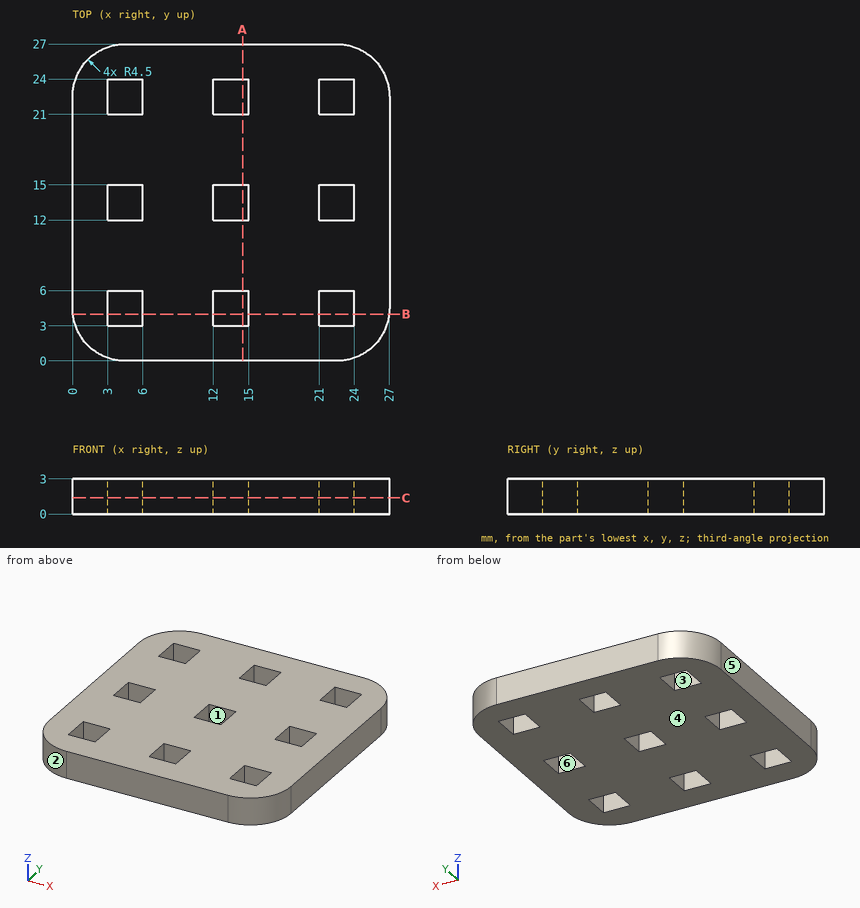
Input: dimensioned drawing with shaded views. Units: mm. Origin: part minimum x, y, z. A direction names the side the tool comes from. Coordinates: 2 decimals unless noted, no trailing zeros. Order: outer loops, then holes, each group sorted by start corner. A loop starts at its lowest first (then second) coordinate and runs counter-clockwise, first axis right, second up. Notation, with made-up numbers: M -37.75,2 L -10.75,2 A21 ccw -10.75,23 Z; hole C -27,-17 d4. An arc over 180 degrees is marked long. Write each question's results on one line, items separated by ' | '. Start each with the question number.
Item 1: First-contact query: pin 1 Ø0.9 at (x, z) = (22, 2) entering from -Y. Flat tip, straight axial feed; report the tip coordinate or a pass-through.
Item 2: Line query: probe 1 along X at (y, z) = (4.5, 1.1); probe 2 along Y at (x, z) = (3.75, 0.2). Output: solid intervals per line, ascending.
Item 3: Cut plane B-B (y = 4). Return loops of the section in (x, z).
Item 4: Cut plane C-C (z = 1.4). Count the separate pieces of the cut face and the enclosed holes in it, and give its area (3 significant figures).
Item 5: Draft query along X for the marked faces 1, 2, 3 and 4. Return one class per face: pulls with the +X half, pulls with the -X half, needs draft (parallel to the pull), parting line crosses it, or undercut.
Item 6: Set-up query: the marked faces 5 and 6. Return all of +Z, -Z, +X, -X, +Y, -Y with unobstructed straight access to the full face (end or side cutting, diameter ignored); none if empty.
Item 7: Cut plane A-A (x = 14.5). Return loops of the section in (y, z), and give its area (3 significant figures).
Checked values:
1) pin 1: stops at y = 0
2) probe 1: x = 0 to 3, 6 to 12, 15 to 21, 24 to 27 | probe 2: y = 0.06 to 3, 6 to 12, 15 to 21, 24 to 26.94
3) outline: M 0.03,0 L 3,0 L 3,3 L 0.03,3 Z; M 6,0 L 12,0 L 12,3 L 6,3 Z; M 15,0 L 21,0 L 21,3 L 15,3 Z; M 24,0 L 26.97,0 L 26.97,3 L 24,3 Z
4) separate pieces: 1 | enclosed holes: 9 | area: 631 mm2
5) face 1: undercut | face 2: pulls with the -X half | face 3: undercut | face 4: needs draft
6) face 5: +Z, -Z, -X, +Y, -Y | face 6: +Z, -Z
7) outline: M 0,0 L 3,0 L 3,3 L 0,3 Z; M 6,0 L 12,0 L 12,3 L 6,3 Z; M 15,0 L 21,0 L 21,3 L 15,3 Z; M 24,0 L 27,0 L 27,3 L 24,3 Z | area: 54.0 mm2
